from build123d import *

# Parameters (mm, degrees)
SKETCH1_R           = 10
SKETCH1_R_2         = 1
BOSS_EXTRUDE1_DEPTH = 5
FILLET1_R           = 1
FILLET2_R           = 0.2


with BuildPart() as part:
    # Sketch1 → Boss-Extrude1 (new body)
    with BuildSketch(Plane(origin=(0, 0, 0), x_dir=(1, 0, 0), z_dir=(0, 1, 0))):
        with Locations(Location((0, 0, 0), (0, 0, 270))):
            Circle(SKETCH1_R)
        with Locations(Location((-4.372934276, 2.268231964, 0), (0, 0, 270))):
            Circle(SKETCH1_R_2, mode=Mode.SUBTRACT)
        with Locations(Location((4.372934276, 2.268231964, 0), (0, 0, 270))):
            Circle(SKETCH1_R_2, mode=Mode.SUBTRACT)
        with Locations(Location((0, -5.30591238, 0), (0, 0, 270))):
            Circle(SKETCH1_R_2, mode=Mode.SUBTRACT)
    extrude(amount=BOSS_EXTRUDE1_DEPTH)

    # Fillet1
    fillet1_edges = [part.edges().sort_by_distance(p)[0] for p in [
        (0, 5, -10),
    ]]
    fillet(fillet1_edges, radius=FILLET1_R)

    # Fillet2
    fillet2_edges = [part.edges().sort_by_distance(p)[0] for p in [
        (0, 5, 4.30591238),
        (4.372934276, 5, -3.268231964),
        (-4.372934276, 5, -3.268231964),
    ]]
    fillet(fillet2_edges, radius=FILLET2_R)


solid = part.part
Work out the finished part from the listing and answer in its coordinate system (mm). Coordinates: 2 decimals unless noted, no trailing zeros. Loops run counter-clockwise (first coordinate to the right, second up) from the corner with the lowest first, then second, coordinate; pieces in that order, holes last. Notation, with made-up numbers: (-20.5, 4) -> (33.5, 4) arc R33 ccw to (33.5, 38) -> close; hole circle Ø7 at (13.25, 87.25). An arc over 180 degrees is marked (long way). Write each question's results on one line, items separated by ' | '. Start each with the question number.
1) Find section A-A on x = 0. Determine the outline of the cut face in (y, z), then the cut area to 3 significant figures.
2) Find section B-B on z = -2.75. Count the separate pieces of the cut face and the enclosed holes in it, then the cut area to 3 significant figures.
3) The mould has two halves that part along Z. Classify faces 1 (the cylindrical face through (-0.38, 2.37, 6.23)), 2 (the flat face through (0, 0, 0)), 3 (the cylindrical face through (-9.76, 1.97, -2.17)): pulls with the +Z half, pulls with the -Z half, needs draft (parallel to the pull), parting line crosses it, or undercut.
4) Flat-ended cylindrical pins translate along their axes: P1, Ø1.5, axis at y = 4.5, z = 7.5, coming from the +X side; P2, Ø1.5, axis at x = -7.5, y = 3.5, coming from the +Z side; P3, Ø1.5, axis at y = 3.5, z = -4, coming from the -X side; P4, Ø1.2, axis at x = 0, z = 5.31, coming from the +Y side. Find the tip coordinate at first contact, or state that the pin passes through.
5) Consider line 1 along X through (y, z) = (2.6, 6); line 2 along X through (y, z) = (1.7, 5.75); line 3 along Z through (x, y) = (-3.75, 1.3). Determine where each line is inside the solid, lowest interval first.
6) Find section C-C on y = 1.7. Determine the outline of the cut face in (x, z), then the cut area to 3 significant figures.
Response values:
1) outline: (0, -10) -> (4, -10) arc R1 ccw to (5, -9) -> (5, 4.11) arc R0.2 ccw to (4.8, 4.31) -> (0, 4.31) -> close; (0, 6.31) -> (4.8, 6.31) arc R0.2 ccw to (5, 6.51) -> (5, 9) arc R1 ccw to (4, 10) -> (0, 10) -> close | area: 89.6 mm^2
2) separate pieces: 3 | enclosed holes: 0 | area: 78.1 mm^2
3) face 1: undercut | face 2: needs draft | face 3: parting line crosses it
4) P1: stops at x = 7.3 | P2: stops at z = 7.38 | P3: stops at x = -9.46 | P4: passes through
5) line 1: x = -8 to -0.72, 0.72 to 8 | line 2: x = -8.18 to -0.9, 0.9 to 8.18 | line 3: z = -9.27 to -3.05, -1.49 to 9.27
6) outline: circle Ø20 at (0, 0); hole circle Ø2 at (-4.37, -2.27); hole circle Ø2 at (0, 5.31); hole circle Ø2 at (4.37, -2.27) | area: 305 mm^2
